```python
from build123d import *

# Parameters (mm, degrees)
F1_DEPTH    = 4.0000047
F2_T1_DEPTH = 112.2565983155
F3_T1_DEPTH = 247.2565983155


# Not quite as in the source:
# - a fillet or chamfer that OpenCascade refuses, or shapes differently, is made with other operations: its cross-section is extruded or revolved along the edge and cut away or added


with BuildPart() as f1:
    # F0 (on Right) → F1 (new body, symmetric)
    with BuildSketch(Plane.YZ):
        Polygon((-99.9751089393, -29.498891169), (-99.9751089393, -89.4988911689), (95.0248910607, -89.4988911689), (95.0248910607, 105.5011088311), align=None)
    extrude(amount=F1_DEPTH, both=True)

    # F2: chamfer of 10.16 on 1 edges, made by hand

    # F2_s2 → F2_t1 (cut)
    with BuildSketch(Plane.XY.offset(-115.6271903267)):
        Polygon((6.1599953, -99.9751089393), (-4.0000047, -89.8151089393), (-4.0000047, -99.9751089393), align=None)
    extrude(amount=F2_T1_DEPTH, mode=Mode.SUBTRACT)

    # F3: chamfer of 10.16 on 1 edges, made by hand

    # F3_s2 → F3_t1 (cut)
    with BuildSketch(Plane.XY.offset(-115.6271903267)):
        Polygon((-4.0000047, 84.8648910607), (6.1599953, 95.0248910607), (-4.0000047, 95.0248910607), align=None)
    extrude(amount=F3_T1_DEPTH, mode=Mode.SUBTRACT)


solid = f1.part
```
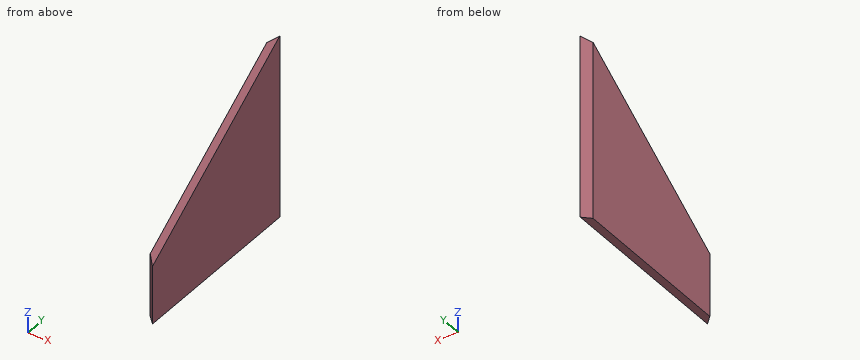
Check sheet for the modelled part. Datum: model origin and axes. Units: mm. Give positions to 0.01 mm unless a question says otherwise; leave off trailing zeros. Write each loop counter-clockwise with the first axis right and the second up, starting at its lowest first coordinate (ties: lowest second). Pieces come first, ordered by that corner, then holes.
Item 1: Cross-section at B-B (x = -0.5). Enter the section's corners in (y, z), and give its area (3 significant figures).
Item 2: Gauge pin test, flat ends, axial feed: pin 1 (1 mm diameter, centred on x = 2, z = -17, fed in from -Y); pin 2 (4 mm diameter, centred on x = 0.5, z = -62.5, fed in from +Y); pin 3 (4 mm diameter, centred on x = 3, z = -7.5, fed in from +Y). Record the tip position at first contact, or that the pin passes through.
Item 3: Scan lines: L1, parallel to Y at x = 2, z = 91; L2, parallel to Y at x = 3.25, z = -60.5; L3, parallel to Z at x = 2.5, y = -14. Record each from-to range of solid material in increasing order.
Item 4: Cross-section at A-A (z = -52). Enter the section's corners in (x, y).
Report:
1. outline: (-93.32, -89.5) - (88.36, -89.5) - (88.36, 100.89) - (-93.32, -24.89) - close
1. area: 23,200 mm2
2. pin 1: stops at y = -82.64
2. pin 2: stops at y = 91.36
2. pin 3: stops at y = 92.86
3. L1: y = 74.08 to 90.86
3. L2: y = -97.07 to 92.11
3. L3: z = -89.5 to 30.02
4. outline: (-4, -89.82) - (4, -97.82) - (4, 92.86) - (-4, 84.86) - close
